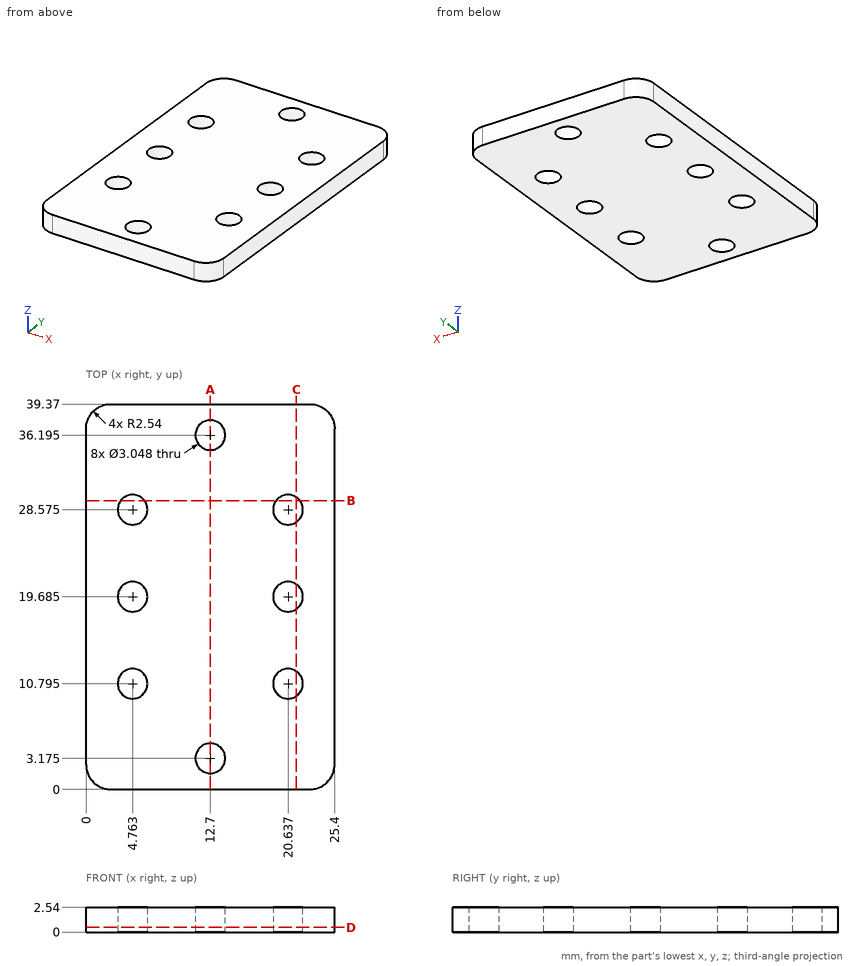
The figure shows three views and two pictorial views of one solid part (mm, origin at its lowest corner). Answer the questions. Coordinates: 2 decimals unless noted, no trailing zeros. Write each loop counter-clockwise with the first axis right and the second up, starting at its lowest first coordinate (ties: lowest second). Pieces come first, ordered by that corner, then holes. Notation, with made-up numbers: (5, -3) -> (33, -3) arc R25 ccw to (33, 35) -> close; hole circle Ø2 at (17, 11.25). An arc over 180 degrees is marked (long way). Answer as a JSON object with one key per item and string values.
Q1. Consider line 1 (Y direction, x = 12.7, z = 1.7); line 2 (X direction, y = 18.5, z = 0.15) (1 decimal); line 3 (X direction, y = 11, z = 1.05). Determine where each line is inside the solid, lowest interval first. Write a range as [from, to].
The answers:
{"line 1": "y = [0, 1.65], [4.7, 34.67], [37.72, 39.37]", "line 2": "x = [0, 3.8], [5.7, 19.7], [21.6, 25.4]", "line 3": "x = [0, 3.25], [6.27, 19.13], [22.15, 25.4]"}
Q2. A flat-ended cylindrical pin translates along its axis: pin 1 Ø3.5 at (x, y) = (4.76, 19.68) entering from -Z. Find the tip coordinate at first contact, or state that the pin passes through.
The answers:
{"pin 1": "stops at z = 0"}
Q3. The part is cut by section A-A on x = 12.7. Give the vertices of the cut face in (y, z).
The answers:
{"outline": "(0, 0) -> (1.65, 0) -> (1.65, 2.54) -> (0, 2.54) -> close; (4.7, 0) -> (34.67, 0) -> (34.67, 2.54) -> (4.7, 2.54) -> close; (37.72, 0) -> (39.37, 0) -> (39.37, 2.54) -> (37.72, 2.54) -> close"}
Q4. The part is cut by section C-C on x = 21.5. Give the vertices of the cut face in (y, z).
The answers:
{"outline": "(0, 0) -> (9.54, 0) -> (9.54, 2.54) -> (0, 2.54) -> close; (12.05, 0) -> (18.43, 0) -> (18.43, 2.54) -> (12.05, 2.54) -> close; (20.94, 0) -> (27.32, 0) -> (27.32, 2.54) -> (20.94, 2.54) -> close; (29.83, 0) -> (39.37, 0) -> (39.37, 2.54) -> (29.83, 2.54) -> close"}
Q5. The part is cut by section D-D on z = 0.5. Give the number of separate pieces and of enclosed holes in the cut face, then the cut area to 3 significant figures.
The answers:
{"separate pieces": "1", "enclosed holes": "8", "area": "936 mm2"}
Q6. The part is cut by section B-B on y = 29.5. Give the vertices of the cut face in (x, z).
The answers:
{"outline": "(0, 0) -> (3.55, 0) -> (3.55, 2.54) -> (0, 2.54) -> close; (5.97, 0) -> (19.43, 0) -> (19.43, 2.54) -> (5.97, 2.54) -> close; (21.85, 0) -> (25.4, 0) -> (25.4, 2.54) -> (21.85, 2.54) -> close"}
